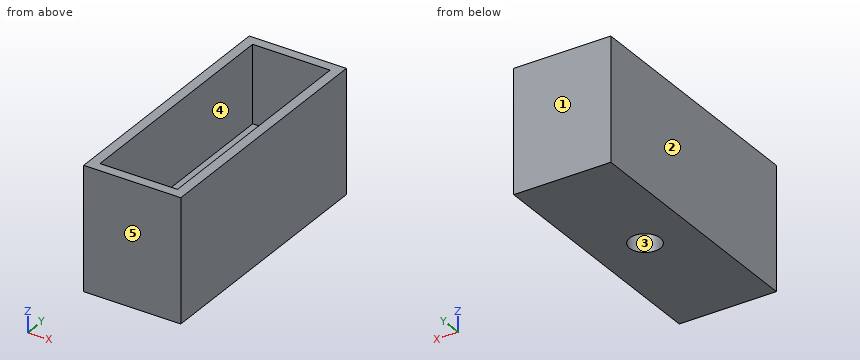
from build123d import *

# Parameters (mm, degrees)
SKETCH_W        = 7.9
SKETCH_H        = 20.6
PAD_DEPTH       = 10
SKETCH001_W     = 6.3
SKETCH001_H     = 19
POCKET_DEPTH    = 6.3
SKETCH003_R     = 1.25
POCKET001_DEPTH = 10


with BuildPart() as part:
    # Sketch → Pad (new body)
    with BuildSketch(Plane.XY):
        Rectangle(SKETCH_W, SKETCH_H)
    extrude(amount=PAD_DEPTH)

    # Sketch001 (on Face6 of Pad) → Pocket (cut)
    with BuildSketch(Plane.XY.offset(10)):
        Rectangle(SKETCH001_W, SKETCH001_H)
    extrude(amount=-POCKET_DEPTH, mode=Mode.SUBTRACT)

    # Sketch003 (on Face5 of Pocket) → Pocket001 (cut)
    with BuildSketch(Plane.XY.offset(10)):
        Circle(SKETCH003_R)
    extrude(amount=-POCKET001_DEPTH, mode=Mode.SUBTRACT)


solid = part.part
Build history of the part. All positions in model axes, mm. Face numbers are marked on the shaded views. A direction names the side the tool comes from. Round coordinates to 2 decimals unless told otherwise and drop trailing zeros. Loops run counter-clockwise (first coordinate to the right, second up) from the corner with the lowest first, then second, coordinate; pieces in that order, holes last. Notation, with made-up numbers: (86.25, 16) -> (126.25, 16) arc R19 ccw to (126.25, 32) -> close; hole circle Ø5 at (60.25, 51). An arc over 180 degrees is marked (long way). Use CSV: the item, a comma, the result in double quotes. Start each with the question number.
Q1. Drill centre lines: L1, parallel to Y at x = -0.5, z = 9; L2, parallel to X at y = -2.25, z = 8.5; L3, parallel to Y at x = 0, z = 2.45. Where is each one in solid material? Low to high.
Q2. Flat gauge pin, fed straight in: pin 1 Ø1.9 at (x, y) = (-1.5, 0.5) entering from +Z. Where does the tip first touch, or does it go through?
Q3. Saw through at C-C on y = 0. Give the cut face in (x, z), and give its area (3 significant figures).
Q4. Saw through at B-B on x = 0.75. Give the cut face in (y, z).
Q5. Which spindle directions (+Z, -Z, +X, -X, +Y, -Y) get a long thin tool onto all of the face, cutting with end or side? Do the marked faces 4 and 5. Say none if no direction does.
Q6. Saw through at A-A on z = 8.5. Give the cut face in (x, y), and give its area (3 significant figures).
Q7. Mould opens along X. For the marked faces 1, 2 and 3 say: +X half, -X half, draft (parallel to the pull), parting line (faces both ways), or undercut.
Solutions:
1,L1,"y = -10.3 to -9.5, 9.5 to 10.3"
1,L2,"x = -3.95 to -3.15, 3.15 to 3.95"
1,L3,"y = -10.3 to -1.25, 1.25 to 10.3"
2,pin 1,"stops at z = 3.7"
3,outline,"(-3.95, 0) -> (-1.25, 0) -> (-1.25, 3.7) -> (-3.15, 3.7) -> (-3.15, 10) -> (-3.95, 10) -> close; (1.25, 0) -> (3.95, 0) -> (3.95, 10) -> (3.15, 10) -> (3.15, 3.7) -> (1.25, 3.7) -> close"
3,area,"30.1 mm^2"
4,outline,"(-10.3, 0) -> (-1, 0) -> (-1, 3.7) -> (-9.5, 3.7) -> (-9.5, 10) -> (-10.3, 10) -> close; (1, 0) -> (10.3, 0) -> (10.3, 10) -> (9.5, 10) -> (9.5, 3.7) -> (1, 3.7) -> close"
5,face 4,"+Z"
5,face 5,"+Z, -Z, +X, -X, -Y"
6,outline,"(-3.95, -10.3) -> (3.95, -10.3) -> (3.95, 10.3) -> (-3.95, 10.3) -> close; hole (-3.15, -9.5) -> (3.15, -9.5) -> (3.15, 9.5) -> (-3.15, 9.5) -> close"
6,area,"43.0 mm^2"
7,face 1,"draft"
7,face 2,"-X half"
7,face 3,"undercut"
